```python
from build123d import *

# Parameters (mm, degrees)
ESQUISSE1_W             = 40
ESQUISSE1_H             = 20
BOSS_EXTRU_1_DEPTH      = 5
CONG_1_R                = 3
ESQUISSE2_R             = 0.79
ENL_V_MAT_EXTRU_1_DEPTH = 46


with BuildPart() as part:
    # Esquisse1 → Boss.-Extru.1 (new body)
    with BuildSketch(Plane.XY):
        with Locations((20, 10)):
            Rectangle(ESQUISSE1_W, ESQUISSE1_H)
    extrude(amount=BOSS_EXTRU_1_DEPTH)

    # Congé1
    cong_1_edges = [part.edges().sort_by_distance(p)[0] for p in [
        (0, 20, 2.5),
        (40, 20, 2.5),
        (40, 0, 2.5),
        (0, 0, 2.5),
    ]]
    fillet(cong_1_edges, radius=CONG_1_R)

    # Esquisse2 → Enlèv. mat.-Extru.1 (cut, through all)
    with BuildSketch(Plane.XY.offset(5)):
        with Locations((5, 17.5)):
            Circle(ESQUISSE2_R)
        with Locations((5, 2.5)):
            Circle(ESQUISSE2_R)
        with Locations((17.5, 2.5)):
            Circle(ESQUISSE2_R)
        with Locations((17.5, 17.5)):
            Circle(ESQUISSE2_R)
        with Locations(Location((22.5, 17.5, 0), (0, 0, 180))):
            Circle(ESQUISSE2_R)
        with Locations(Location((22.5, 2.5, 0), (0, 0, 180))):
            Circle(ESQUISSE2_R)
        with Locations(Location((35, 2.5, 0), (0, 0, 180))):
            Circle(ESQUISSE2_R)
        with Locations(Location((35, 17.5, 0), (0, 0, 180))):
            Circle(ESQUISSE2_R)
    extrude(amount=-ENL_V_MAT_EXTRU_1_DEPTH, mode=Mode.SUBTRACT)


solid = part.part
```
Model file for the job. Use its own axes, mm. Coordinates: 2 decimals unless noted, no trailing zeros. Write each loop counter-clockwise with the first axis right and the second up, starting at its lowest first coordinate (ties: lowest second). Pieces come first, ordered by that corner, then holes. Notation, with made-up numbers: (70, 82) - (100, 82) arc R20 ccw to (100, 89) - close; hole circle Ø6 at (-6, 75.25). An arc over 180 degrees is marked (long way). One line per item, written item: value. Start each with the question number.
1. Mould opens along X. For faces 1 (the flat face through (20, 0, 2)), 2 (the cylindrical face through (39.14, 19.1, 2.54)), 3 (the cylindrical face through (4.373, 17.019, 2.535)) say: released by +X, released by -X, zero draft, split by the parting line, or undercut.
2. Slice it at C-C (y = 2.5). Write the cut outline in (x, z), plus the area to 3 significant figures.
3. Slice it at B-B (z = 1.95). Count the separate pieces of the cut face and the enclosed holes in it, plus the area to 3 significant figures.
4. Probe line 1 (Y direction, x = 22.5, z = 3.75); line 2 (Y direction, x = 35.5, z = 1.45); line 3 (X direction, y = 17, z = 3.2). List the from-to ranges inside material, lowest first. Write a range as from..to.
5. Flat gauge pins, fed straight in: pin 1 (1.4 mm diameter, centred on x = 5, y = 2.5, fed in from +Z); pin 2 (1.8 mm diameter, centred on x = 22.5, y = 17.5, fed in from +Z). Where does each tip first touch, or does it go through?
6. Slice it at A-A (x = 22.5). Write the cut outline in (y, z).
Answers below:
1. face 1: zero draft
1. face 2: released by +X
1. face 3: undercut
2. outline: (0.04, 0) - (4.21, 0) - (4.21, 5) - (0.04, 5) - close; (5.79, 0) - (16.71, 0) - (16.71, 5) - (5.79, 5) - close; (18.29, 0) - (21.71, 0) - (21.71, 5) - (18.29, 5) - close; (23.29, 0) - (34.21, 0) - (34.21, 5) - (23.29, 5) - close; (35.79, 0) - (39.96, 0) - (39.96, 5) - (35.79, 5) - close
2. area: 168 mm^2
3. separate pieces: 1
3. enclosed holes: 8
3. area: 777 mm^2
4. line 1: y = 0..1.71, 3.29..16.71, 18.29..20
4. line 2: y = 0..1.89, 3.11..16.89, 18.11..20
4. line 3: x = 0..4.39, 5.61..16.89, 18.11..21.89, 23.11..34.39, 35.61..40
5. pin 1: passes through
5. pin 2: stops at z = 5
6. outline: (0, 0) - (1.71, 0) - (1.71, 5) - (0, 5) - close; (3.29, 0) - (16.71, 0) - (16.71, 5) - (3.29, 5) - close; (18.29, 0) - (20, 0) - (20, 5) - (18.29, 5) - close
